Check sheet for the modelled part. Datum: model origin and axes. Units: mm. A direction names the side the tool comes from. Give positions to 0.01 mm unless a question says otherwise; leave off trailing zeros. Write each loop counter-clockwise with the first axis right and the second up, starting at its lowest first coordinate (ties: lowest second). Pieces come first, ordered by that corner, then holes. Notation, with made-up numbers: (-14, 55) -> (23, 55) arc R10 cw to (23, 65) -> close; hole circle Ø4 at (54, 47.5). An arc over 180 degrees is marked (long way). Use a Markdown table: item, result. Add a question column.
1. Cross-section at C-C (z = 4.6). Enter the section's corners in (x, y).
2. Release check for a two-part mould opening along X. For faces 1 (the cylindrical face through (3.4, 6.2, 2.5)), 2 (the flat face through (10, 6, 2)), 3 (the flat face through (5, 14, 2)) record: released by +X, released by -X, zero draft, split by the parting line, or undercut.
3. Gauge pin test, flat ends, axial feed: P1, Ø1, axis at x = 4, z = 0.5, coming from the +Y side; P2, Ø1.5, axis at x = 4.5, y = 11.5, coming from the -Z side. Record the tip position at first contact, or that the pin passes through.
4. Cross-section at B-B (y = 5). Enter the section's corners in (x, z).
5. Set-up check for faces 4 (the flat face through (5, 11, 2)), 5 (the flat face through (7.2, 5.1, 0)): record each of +Z, -Z, +X, -X, +Y, -Y from which the full face is reachable in a straight line by a thin tool's end or side.
6. Scan lines: probe 1 along X at (y, z) = (5, 2.65); probe 2 along Y at (x, z) = (5, 3.15). Record each from-to range of solid material in increasing order. Write a range as [from, to].
7. Cross-section at D-D (x = 2.25). Enter the section's corners in (y, z), then the cut area to 3 significant figures.
8. Cross-section at A-A (x = 5). Enter the section's corners in (y, z).
from build123d import *

# Parameters (mm, degrees)
F0_W     = 10
F0_H     = 15
F1_DEPTH = 5
F2_W     = 5
F2_H     = 2
F3_DEPTH = 25
F4_R     = 2
F5_DEPTH = 25
F6_W     = 10
F6_H     = 0.791458
F7_DEPTH = 0.3


with BuildPart() as f1:
    # F0 (on Top) → F1 (new body)
    with BuildSketch(Plane.XY):
        with Locations((5, 7.5)):
            Rectangle(F0_W, F0_H)
    extrude(amount=F1_DEPTH)

    # F2 (on face) → F3 (cut)
    with BuildSketch(Plane.YZ.offset(10)):
        with Locations((12.5, 1)):
            Rectangle(F2_W, F2_H)
    extrude(amount=-F3_DEPTH, mode=Mode.SUBTRACT)

    # F4 (on face) → F5 (cut)
    with BuildSketch(Plane(origin=(0, 0, 0), x_dir=(1, 0, 0), z_dir=(0, 0, -1))):
        with Locations((5, -5)):
            Circle(F4_R)
    extrude(amount=-F5_DEPTH, mode=Mode.SUBTRACT)

    # F6 (on face) → F7 (join)
    with BuildSketch(Plane(origin=(0, 0, 2), x_dir=(1, 0, 0), z_dir=(0, 0, -1))):
        with Locations((5, -13.373503)):
            Rectangle(F6_W, F6_H)
    extrude(amount=F7_DEPTH)


solid = f1.part
Worked answers:
| question | item | result |
|---|---|---|
| 1 | outline | (0, 0) -> (10, 0) -> (10, 15) -> (0, 15) -> close; hole circle Ø4 at (5, 5) |
| 2 | face 1 | undercut |
| 2 | face 2 | released by +X |
| 2 | face 3 | zero draft |
| 3 | P1 | stops at y = 10 |
| 3 | P2 | stops at z = 2 |
| 4 | outline | (0, 0) -> (3, 0) -> (3, 5) -> (0, 5) -> close; (7, 0) -> (10, 0) -> (10, 5) -> (7, 5) -> close |
| 5 | face 4 | -Z, +X, -X |
| 5 | face 5 | -Z, +X, -X, +Y, -Y |
| 6 | probe 1 | x = [0, 3], [7, 10] |
| 6 | probe 2 | y = [0, 3], [7, 15] |
| 7 | outline | (0, 0) -> (10, 0) -> (10, 2) -> (12.98, 2) -> (12.98, 1.7) -> (13.77, 1.7) -> (13.77, 2) -> (15, 2) -> (15, 5) -> (0, 5) -> close |
| 7 | area | 65.2 mm² |
| 8 | outline | (0, 0) -> (3, 0) -> (3, 5) -> (0, 5) -> close; (7, 0) -> (10, 0) -> (10, 2) -> (12.98, 2) -> (12.98, 1.7) -> (13.77, 1.7) -> (13.77, 2) -> (15, 2) -> (15, 5) -> (7, 5) -> close |
